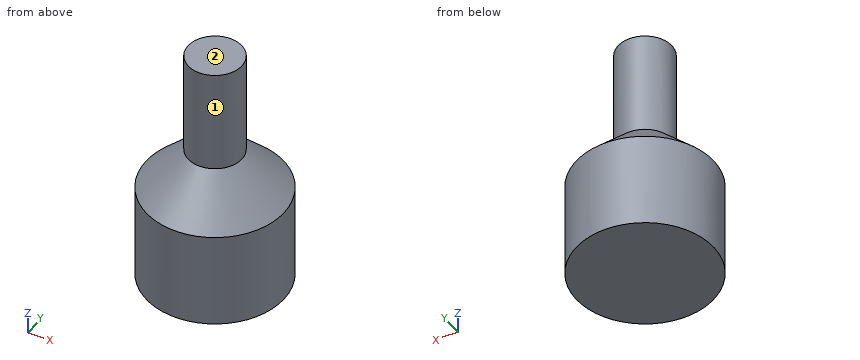
```python
from build123d import *

# Parameters (mm, degrees)
F0_R        = 3.9
F1_DEPTH    = 15
F2_R        = 10
F3_DEPTH    = 20
F4_S5_R     = 3.9
F4_T6_DEPTH = 16


# Not quite as in the source:
# - a fillet or chamfer that OpenCascade refuses, or shapes differently, is made with other operations: its cross-section is extruded or revolved along the edge and cut away or added


with BuildPart() as f1:
    # F0 (on Top) → F1 (new body)
    with BuildSketch(Plane.XY):
        Circle(F0_R)
    extrude(amount=F1_DEPTH)

    # F2 (on Top) → F3 (join)
    with BuildSketch(Plane.XY):
        Circle(F2_R)
    extrude(amount=-F3_DEPTH)

    # F4: chamfer of 6.1 on 1 edges, made by hand


with BuildPart() as f4_tool2:
    # F4_s3 → F4_t4 (revolve)
    with BuildSketch(Plane.XZ):
        Polygon((10, -6.1), (3.9, 0), (10, 0), align=None)
    revolve(axis=Axis((0, 0, 0), (0, 0, 1)))

    # F4_s5 → F4_t6 (cut, symmetric)
    with BuildSketch(Plane.XY.offset(-3)):
        Circle(F4_S5_R)
    extrude(amount=F4_T6_DEPTH, both=True, mode=Mode.SUBTRACT)


with BuildPart() as f1_1:
    add(f1.part)

    # F4_t1: cut F4_tool2
    add(f4_tool2.part, mode=Mode.SUBTRACT)


solid = f1_1.part
```
Could you check a few things on this model? Use its own coordinates, in mm. Face numbers are marked on the shaded views. A direction names the side the tool comes from. Give positions to 0.01 mm unless a question says otherwise; leave off trailing zeros. Write each loop counter-clockwise with the first axis right and the second up, starting at its lowest first coordinate (ties: lowest second). Pieces come first, ordered by that corner, then holes. Notation, with made-up numbers: (-8, 44) - (9, 44) arc R8 cw to (9, 48) - close; hole circle Ø10 at (-3.75, 70). An arc over 180 degrees is marked (long way). One line per item, written item: value. Start each with the question number.
Item 1: Imagine slicing it at C-C, the plane z = -16. List the corners of the cut face in (x, y) for me, and give its area (3 significant figures).
Item 2: Please list where these lines run through material, in increasing order: line 1 (X direction, y = 0.25, z = -16); line 2 (Z direction, x = -7.25, y = -3.5); line 3 (X direction, y = -0.25, z = 6). Write a range as from..to.
Item 3: Imagine slicing it at D-D, the plane z = 0.5. List the corners of the cut face in (x, y) for me, and give its area (3 significant figures).
Item 4: I'm going to push flat-ended pins straight in: pin 1 (1.5 mm diameter, centred on y = 0, z = -3, fed in from +X); pin 2 (6 mm diameter, centred on y = 3, z = 5.5, fed in from -X); pin 3 (6 mm diameter, centred on x = 5, z = 10.5, fed in from +Y); pin 4 (5 mm diameter, centred on y = -7.5, z = 3, fed in from +X). Where does each tip first touch, or does it pass through?
Item 5: Which directions (+Z, -Z, +X, -X, +Y, -Y) give clear straight access to the entire face, cutting with the end or side of a thin tool? Please do the marked faces 1 and 2.
Item 6: Imagine slicing it at A-A, the plane x = 0. List the corners of the cut face in (y, z) for me, and give its area (3 significant figures).
Geometry says:
1. outline: circle Ø20 at (0, 0)
1. area: 314 mm^2
2. line 1: -10..10
2. line 2: -20..-4.15
2. line 3: -3.89..3.89
3. outline: circle Ø7.8 at (0, 0)
3. area: 47.8 mm^2
4. pin 1: x = 7.65
4. pin 2: x = -3.9
4. pin 3: y = 3.35
4. pin 4: through
5. face 1: +Z
5. face 2: +Z, +X, -X, +Y, -Y
6. outline: (-10, -20) - (10, -20) - (10, -6.1) - (3.9, 0) - (3.9, 15) - (-3.9, 15) - (-3.9, 0) - (-10, -6.1) - close
6. area: 480 mm^2
